Build history of the part. All positions in model axes, mm. A direction names the side the tool comes from. Coordinates: 2 decimals unless noted, no trailing zeros. Loops run counter-clockwise (first coordinate to the right, second up) from the corner with the lowest first, then second, coordinate; pieces in that order, holes last.
Item 1: Drill centre lines: line 1 along X through (y, z) = (10.75, 5); line 2 along X through (y, z) = (6, 4.25); line 3 along Y through (x, z) = (18, 7.75). Where is each one in solid material? Low to high.
Item 2: Flat gauge pin, fed straight in: pin 1 (4.5 mm diameter, centred on x = 73, z = 5, fed in from +Y). Where does the tip first touch, or does it go through?
Item 3: 3-axis set-ups, long thin cutter, end or side, ignore diameter. For faces 4 (the face through (0, 31, 5)), 5 (the face through (70.78, 7.6, 6.15)): which of +Z, -Z, +X, -X, +Y, -Y reach the whole face in a straight line?
Item 4: Mould opens along X. For faces 1 (the face through (5, 68, 5)), 2 (the face through (78, 31, 5)), 3 (the face through (5.751, 7.605, 7.385)) say: released by +X, released by -X, zero draft, split by the parting line, or undercut.
Item 5: Cut at B-B (y = 55). List the corners of the cut face in (x, z), and give its area (3 significant figures).
Item 6: Cut at A-A (x = 18). List the corners of the cut face in (y, z), and give its area (3 significant figures).
Item 7: Cut at C-C (x = 60). List the corners of the cut face in (y, z).
Item 8: Cut at D-D (z = 3.75). Count the separate pieces of the cut face and the enclosed holes in it, and give its area (3 significant figures).
from build123d import *
from OCP.BRepFilletAPI import BRepFilletAPI_MakeChamfer

# Parameters (mm, degrees)
SKETCH1_W             = 78
SKETCH1_H             = 73
EXTRUDE1_DEPTH        = 10
SKETCH3_R             = 12.0065
F_24DIA_HOLE_DEPTH    = 108.29864864
M6_TAPPED_HOLE1_D     = 5
M6_TAPPED_HOLE1_DEPTH = 15
M6_TAPPED_HOLE1_TIP   = 1.502151548
SKETCH7_R             = 8.0045
F_16DIA_HOLE_DEPTH    = 108.29864864
CHAMFER1_SIZE         = 10
CHAMFER2_SIZE         = 1.5
CHAMFER2_SIZE2        = 0.401923789
CHAMFER3_SIZE         = 1.5
CHAMFER3_SIZE2        = 0.401923789


with BuildPart() as part:
    # Sketch1 → Extrude1 (new body)
    with BuildSketch(Plane.XY):
        with Locations((39, 36.5)):
            Rectangle(SKETCH1_W, SKETCH1_H)
    extrude(amount=EXTRUDE1_DEPTH)

    # Sketch3 → 24dia Hole (cut, through all)
    with BuildSketch(Plane.XY.offset(10)):
        with Locations((18, 55)):
            Circle(SKETCH3_R)
    extrude(amount=-F_24DIA_HOLE_DEPTH, mode=Mode.SUBTRACT)

    # M6 Tapped Hole1
    with Locations(Plane(origin=(5, 0, 5), x_dir=(0, 0, -1), z_dir=(0, -1, 0))):
        with Locations((0, 0), (0, 68), (1.921473379, -8.468632325)):
            Hole(M6_TAPPED_HOLE1_D / 2, depth=M6_TAPPED_HOLE1_DEPTH)
            with Locations((0, 0, -(M6_TAPPED_HOLE1_DEPTH + M6_TAPPED_HOLE1_TIP / 2))):  # 118° drill point
                Cone(0, M6_TAPPED_HOLE1_D / 2, M6_TAPPED_HOLE1_TIP, mode=Mode.SUBTRACT)

    # Sketch7 → 16dia hole (cut, through all)
    with BuildSketch(Plane.XY.offset(10)):
        with Locations((60, 55)):
            Circle(SKETCH7_R)
    extrude(amount=-F_16DIA_HOLE_DEPTH, mode=Mode.SUBTRACT)

    # Chamfer1
    chamfer1_edges = [part.edges().sort_by_distance(p)[0] for p in [
        (0, 73, 5),
        (78, 73, 5),
    ]]
    chamfer(chamfer1_edges, length=CHAMFER1_SIZE)

    # Chamfer2: one chamfer whose edges measure the first distance from different faces: ONE call of the kernel's chamfer builder (chamfer() names one face for all edges)
    chamfer2_edges_1 = [part.edges().sort_by_distance(p)[0] for p in [
        (5.9935, 55, 0),
    ]]
    chamfer2_side_1 = [part.faces().sort_by_distance(p)[0] for p in [
        (5.9935, 55, 5),
    ]]
    chamfer2_edges_2 = [part.edges().sort_by_distance(p)[0] for p in [
        (51.9955, 55, 0),
    ]]
    chamfer2_side_2 = [part.faces().sort_by_distance(p)[0] for p in [
        (51.9955, 55, 5),
    ]]
    chamfer2 = BRepFilletAPI_MakeChamfer(part.part.solid().wrapped)
    for e in chamfer2_edges_1:
        chamfer2.Add(CHAMFER2_SIZE, CHAMFER2_SIZE2, e.wrapped, chamfer2_side_1[0].wrapped)  # the first distance lies on this face
    for e in chamfer2_edges_2:
        chamfer2.Add(CHAMFER2_SIZE, CHAMFER2_SIZE2, e.wrapped, chamfer2_side_2[0].wrapped)  # the first distance lies on this face
    add(Compound.cast(chamfer2.Shape()), mode=Mode.REPLACE)

    # Chamfer3
    chamfer3_edges = [part.edges().sort_by_distance(p)[0] for p in [
        (51.9955, 55, 10),
    ]]
    chamfer3_side = [part.faces().sort_by_distance(p)[0] for p in [
        (51.9955, 55, 5.75),
    ]]
    chamfer(chamfer3_edges, length=CHAMFER3_SIZE, length2=CHAMFER3_SIZE2, reference=chamfer3_side[0])


solid = part.part
Filled sheet:
1. line 1: x = 0 to 2.5, 7.5 to 70.5, 75.5 to 78
1. line 2: x = 0 to 2.62, 7.38 to 70.62, 75.38 to 78
1. line 3: y = 0 to 42.99, 67.01 to 73
2. pin 1: stops at y = 70.25
3. face 4: +Z, -Z, -X, +Y, -Y
3. face 5: -Y
4. face 1: released by -X
4. face 2: released by +X
4. face 3: undercut
5. outline: (0, 0) - (5.59, 0) - (5.99, 1.5) - (5.99, 10) - (0, 10) - close; (30.01, 1.5) - (30.41, 0) - (51.59, 0) - (52, 1.5) - (52, 8.5) - (51.59, 10) - (30.01, 10) - close; (68, 1.5) - (68.41, 0) - (78, 0) - (78, 10) - (68.41, 10) - (68, 8.5) - close
5. area: 378 mm2
6. outline: (0, 0) - (42.59, 0) - (42.99, 1.5) - (42.99, 10) - (0, 10) - close; (67.01, 1.5) - (67.41, 0) - (73, 0) - (73, 10) - (67.01, 10) - close
6. area: 489 mm2
7. outline: (0, 0) - (46.59, 0) - (47, 1.5) - (47, 8.5) - (46.59, 10) - (0, 10) - close; (63, 1.5) - (63.41, 0) - (73, 0) - (73, 10) - (63.41, 10) - (63, 8.5) - close
8. separate pieces: 1
8. enclosed holes: 2
8. area: 4,810 mm2
